For this review, take the finished solid that the model builds, in its own axes (mm). Face numbers are marked on the shaded views. A direction names the side the tool comes from. Coordinates: 2 decimals unless noted, no trailing zeros. Loops run counter-clockwise (first coordinate to the right, second up) from the corner with the lowest first, then second, coordinate; pieces in that order, holes last. Notation, with made-up numbers: M 34,-19 L 52,-19 A32 cw 52,12 Z; hole C 6,-35.5 d7. An arc over 180 degrees is marked long. Put each result on its own line as item: value.
```python
from build123d import *

# Parameters (mm, degrees)
SKETCH2_R           = 1.5
SKETCH2_W           = 75
SKETCH2_H           = 25
BOSS_EXTRUDE1_DEPTH = 15
FILLET3_R           = 4
FILLET4_R           = 4
FILLET5_R           = 4
FILLET6_R           = 4
FILLET7_R           = 4
FILLET8_R           = 4
FILLET9_R           = 4
FILLET10_R          = 4
SKETCH3_R           = 2.5
CUT_EXTRUDE1_DEPTH  = 10
SKETCH5_W           = 80
SKETCH5_H           = 36
CUT_EXTRUDE2_DEPTH  = 5


with BuildPart() as part:
    # Sketch2 → Boss-Extrude1 (new body)
    with BuildSketch(Plane(origin=(0, 0, 0), x_dir=(1, 0, 0), z_dir=(0, 1, 0))):
        with BuildLine():
            ThreePointArc((-43.5, 22.5), (-50.328427125, 25.328427125), (-47.5, 18.5))
            Line((-47.5, 18.5), (-47.5, -18.5))
            ThreePointArc((-47.5, -18.5), (-50.328427125, -25.328427125), (-43.5, -22.5))
            Line((-43.5, -22.5), (43.5, -22.5))
            ThreePointArc((43.5, -22.5), (50.328427125, -25.328427125), (47.5, -18.5))
            Line((47.5, -18.5), (47.5, 18.5))
            ThreePointArc((47.5, 18.5), (50.328427125, 25.328427125), (43.5, 22.5))
            Line((43.5, 22.5), (-43.5, 22.5))
        make_face()
        with Locations(Location((-47.5, 22.5, 0), (0, 0, 270))):
            Circle(SKETCH2_R, mode=Mode.SUBTRACT)
        with Locations(Location((-47.5, -22.5, 0), (0, 0, 270))):
            Circle(SKETCH2_R, mode=Mode.SUBTRACT)
        Rectangle(SKETCH2_W, SKETCH2_H, mode=Mode.SUBTRACT)
        with Locations(Location((47.5, 22.5, 0), (0, 0, 270))):
            Circle(SKETCH2_R, mode=Mode.SUBTRACT)
        with Locations(Location((47.5, -22.5, 0), (0, 0, 270))):
            Circle(SKETCH2_R, mode=Mode.SUBTRACT)
    extrude(amount=BOSS_EXTRUDE1_DEPTH)

    # Fillet3
    fillet3_edges = [part.edges().sort_by_distance(p)[0] for p in [
        (-43.5, 7.5, -22.5),
    ]]
    fillet(fillet3_edges, radius=FILLET3_R)

    # Fillet4
    fillet4_edges = [part.edges().sort_by_distance(p)[0] for p in [
        (-47.5, 7.5, -18.5),
    ]]
    fillet(fillet4_edges, radius=FILLET4_R)

    # Fillet5
    fillet5_edges = [part.edges().sort_by_distance(p)[0] for p in [
        (47.5, 7.5, -18.5),
    ]]
    fillet(fillet5_edges, radius=FILLET5_R)

    # Fillet6
    fillet6_edges = [part.edges().sort_by_distance(p)[0] for p in [
        (43.5, 7.5, -22.5),
    ]]
    fillet(fillet6_edges, radius=FILLET6_R)

    # Fillet7
    fillet7_edges = [part.edges().sort_by_distance(p)[0] for p in [
        (47.5, 7.5, 18.5),
    ]]
    fillet(fillet7_edges, radius=FILLET7_R)

    # Fillet8
    fillet8_edges = [part.edges().sort_by_distance(p)[0] for p in [
        (43.5, 7.5, 22.5),
    ]]
    fillet(fillet8_edges, radius=FILLET8_R)

    # Fillet9
    fillet9_edges = [part.edges().sort_by_distance(p)[0] for p in [
        (-43.5, 7.5, 22.5),
    ]]
    fillet(fillet9_edges, radius=FILLET9_R)

    # Fillet10
    fillet10_edges = [part.edges().sort_by_distance(p)[0] for p in [
        (-47.5, 7.5, 18.5),
    ]]
    fillet(fillet10_edges, radius=FILLET10_R)

    # Sketch3 → Cut-Extrude1 (cut)
    with BuildSketch(Plane(origin=(0, 15, 0), x_dir=(1, 0, 0), z_dir=(0, 1, 0))):
        with Locations(Location((-47.5, 22.5, 0), (0, 0, 270))):
            Circle(SKETCH3_R)
        with Locations(Location((47.5, 22.5, 0), (0, 0, 270))):
            Circle(SKETCH3_R)
        with Locations(Location((47.5, -22.5, 0), (0, 0, 270))):
            Circle(SKETCH3_R)
        with Locations(Location((-47.5, -22.5, 0), (0, 0, 270))):
            Circle(SKETCH3_R)
    extrude(amount=-CUT_EXTRUDE1_DEPTH, mode=Mode.SUBTRACT)

    # Sketch5 → Cut-Extrude2 (cut)
    with BuildSketch(Plane(origin=(0, 0, 0), x_dir=(-1, 0, 0), z_dir=(0, -1, 0))):
        Rectangle(SKETCH5_W, SKETCH5_H)
    extrude(amount=-CUT_EXTRUDE2_DEPTH, mode=Mode.SUBTRACT)


solid = part.part
```
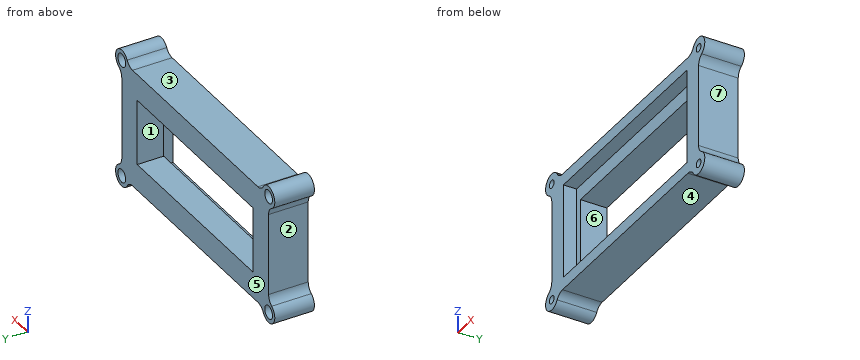
(1) Add section A-A (x = 16.5). Write out the cut boundary in (y, z).
Determined:
outline: M 0,-22.5 L 15,-22.5 L 15,-12.5 L 5,-12.5 L 5,-18 L 0,-18 Z; M 0,18 L 5,18 L 5,12.5 L 15,12.5 L 15,22.5 L 0,22.5 Z
(2) Tool access review of the marked faces 5, 6 and 7: name each direction out of +Z, -Z, +X, -X, +Y, -Y from which nothing blocks a thin tool from reaching the whole face with its end or side.
Determined:
face 5: +Z, -Z, +X, -X, +Y
face 6: +Y, -Y
face 7: +X, +Y, -Y
(3) Add section B-B (y = 10). Write out the cut boundary in (x, z).
Determined:
outline: M -49.5,-19.04 A4 ccw long -44.04,-24.5 A4 cw -40.57,-22.5 L 40.57,-22.5 A4 cw 44.04,-24.5 A4 ccw long 49.5,-19.04 A4 cw 47.5,-15.57 L 47.5,15.57 A4 cw 49.5,19.04 A4 ccw long 44.04,24.5 A4 cw 40.57,22.5 L -40.57,22.5 A4 cw -44.04,24.5 A4 ccw long -49.5,19.04 A4 cw -47.5,15.57 L -47.5,-15.57 A4 cw Z; hole C -47.5,-22.5 d5; hole C -47.5,22.5 d5; hole M -37.5,-12.5 L 37.5,-12.5 L 37.5,12.5 L -37.5,12.5 Z; hole C 47.5,-22.5 d5; hole C 47.5,22.5 d5
(4) Draft analysis for pull direction Z (two halves, no side actions). For the marked faces 1, 2, 3 and 4, state which applies: +Z half, -Z half, draft (parallel to the pull), parting line (faces both ways), or undercut.
Determined:
face 1: undercut
face 2: undercut
face 3: +Z half
face 4: -Z half
(5) Wall thickness on line 1 along Z through (x, y) = (33.5, 6.5); line 2 along X through (y, z) = (2.25, -7); line 3 along X through (y, z) = (2, -17): over which ranges is each line inside the solid? List them lowest first. Write a range as [from, to].
Determined:
line 1: z = [-22.5, -12.5], [12.5, 22.5]
line 2: x = [-47.5, -40], [40, 47.5]
line 3: x = [-47.76, -40], [40, 47.76]
(6) For pin 1 (5.5 mm diameter, centred on x = -13.5, y = 2.5, fed in from +Z); pin 2 (1 mm diameter, centred on y = 4, z = -5.5, fed in from +X); pin 3 (3 mm diameter, centred on x = -0.5, y = 7.5, fed in from -Z), all flat-tipped, find the tip position at first contact; note any pin that passes through.
Determined:
pin 1: stops at z = 22.5
pin 2: stops at x = 47.5
pin 3: stops at z = -22.5
(7) Add section C-C (y = 3.5). Write out the cut boundary in (x, z), plus the area to 3 significant figures.
Determined:
outline: M -49.5,-19.04 A4 ccw long -44.04,-24.5 A4 cw -40.57,-22.5 L 40.57,-22.5 A4 cw 44.04,-24.5 A4 ccw long 49.5,-19.04 A4 cw 47.5,-15.57 L 47.5,15.57 A4 cw 49.5,19.04 A4 ccw long 44.04,24.5 A4 cw 40.57,22.5 L -40.57,22.5 A4 cw -44.04,24.5 A4 ccw long -49.5,19.04 A4 cw -47.5,15.57 L -47.5,-15.57 A4 cw Z; hole C -47.5,-22.5 d3; hole C -47.5,22.5 d3; hole M -40,-18 L 40,-18 L 40,18 L -40,18 Z; hole C 47.5,-22.5 d3; hole C 47.5,22.5 d3
area: 1,530 mm^2
